from build123d import *

# Parameters (mm, degrees)
SKETCH2_W           = 37
SKETCH2_H           = 8
SKETCH2_R           = 2.1
BOSS_EXTRUDE1_DEPTH = 5
SKETCH3_W           = 37
SKETCH3_H           = 5
BOSS_EXTRUDE2_DEPTH = 6
SKETCH4_W           = 37
SKETCH4_H           = 5
BOSS_EXTRUDE3_DEPTH = 57
SKETCH5_W           = 37
SKETCH5_H           = 5
BOSS_EXTRUDE4_DEPTH = 27.5
SKETCH6_R           = 60
BOSS_EXTRUDE5_DEPTH = 5


with BuildPart() as part:
    # Sketch2 → Boss-Extrude1 (new body)
    with BuildSketch(Plane.XY.offset(-2347.018325578)):
        with Locations((0, 1)):
            Rectangle(SKETCH2_W, SKETCH2_H)
        with Locations((10, 1)):
            Circle(SKETCH2_R, mode=Mode.SUBTRACT)
        with Locations((-10, 1)):
            Circle(SKETCH2_R, mode=Mode.SUBTRACT)
    extrude(amount=BOSS_EXTRUDE1_DEPTH)

    # Sketch3 → Boss-Extrude2 (add)
    with BuildSketch(Plane(origin=(0, 5, 0), x_dir=(1, 0, 0), z_dir=(0, 1, 0))):
        with Locations((0, 2344.518325578)):
            Rectangle(SKETCH3_W, SKETCH3_H)
    extrude(amount=BOSS_EXTRUDE2_DEPTH)

    # Sketch4 → Boss-Extrude3 (add)
    with BuildSketch(Plane.XY.offset(-2342.018325578)):
        with Locations((0, 8.5)):
            Rectangle(SKETCH4_W, SKETCH4_H)
    extrude(amount=BOSS_EXTRUDE3_DEPTH)

    # Sketch5 → Boss-Extrude4 (add)
    with BuildSketch(Plane(origin=(0, 11, 0), x_dir=(1, 0, 0), z_dir=(0, 1, 0))):
        with Locations((0, 2287.518325578)):
            Rectangle(SKETCH5_W, SKETCH5_H)
    extrude(amount=BOSS_EXTRUDE4_DEPTH)

    # Sketch6 → Boss-Extrude5 (add)
    with BuildSketch(Plane.XY.offset(-2285.018325578)):
        with Locations((-0.279431791, 76.5)):
            Circle(SKETCH6_R)
    extrude(amount=-BOSS_EXTRUDE5_DEPTH)


solid = part.part
For this review, take the finished solid that the model builds, in its own axes (mm). A direction names the side the tool comes from. Round coordinates to 2 decimals unless told otherwise and drop trailing zeros. Write each loop counter-clockwise with the first axis right and the second up, starting at its lowest first coordinate (ties: lowest second). Pieces come first, ordered by that corner, then holes. Notation, with made-up numbers: (2.25, 82) -> (43.25, 82) arc R9 ccw to (43.25, 98) -> close; hole circle Ø10 at (-1, 29). An arc over 180 degrees is marked (long way). Use CSV: the item, a comma, the result in double quotes.
(1) Consider section A-A, the plane y = 1. Give the boundary of the cut face in (x, z).
Computed values:
outline,"(-18.5, -2347.02) -> (-12.1, -2347.02) -> (-12.1, -2342.02) -> (-18.5, -2342.02) -> close; (-7.9, -2347.02) -> (7.9, -2347.02) -> (7.9, -2342.02) -> (-7.9, -2342.02) -> close; (12.1, -2347.02) -> (18.5, -2347.02) -> (18.5, -2342.02) -> (12.1, -2342.02) -> close"
(2) Consider section C-C, the plane z = -2320.5. Give the boundary of the cut face in (x, y), plus the area to 3 significant figures.
Computed values:
outline,"(-18.5, 6) -> (18.5, 6) -> (18.5, 11) -> (-18.5, 11) -> close"
area,"185 mm²"
(3) Draft analysis for pull direction X (two halves, no side actions). For faces 1 (the face through (-12.1, 1.09, -2344.55)), 2 (the face through (-1, 75, -2290.018)), 3 (the face through (18.5, 9, -2316)), state which applies: +X half, -X half, draft (parallel to the pull), parting line (faces both ways), or undercut.
Computed values:
face 1,"undercut"
face 2,"draft"
face 3,"+X half"
(4) To check wall thickness, follow L1, parallel to Y at x = 10, z = -2345; L2, parallel to Y at x = -18, z = -2330; L3, parallel to Z at x = 42.5, y = 43. State the ranges of each line that lie inside material, in increasing order. Write a range as [from, to].
Computed values:
L1,"[-3, -1.1], [3.1, 11]"
L2,"[6, 11]"
L3,"[-2290.02, -2285.02]"
(5) For faces 4 (the face through (0, 6, -2314)), 5 (the face through (-18.5, 9, -2316)), 6 (the face through (0, 11, -2319)), list the 3-axis set-ups (+Z, -Z, +X, -X, +Y, -Y) from which the entire face can be reached by the end or side of a thin tool; tool diameter is ignored.
Computed values:
face 4,"+Z, +X, -X, -Y"
face 5,"+Z, -Z, -X, -Y"
face 6,"-Z, +X, -X, +Y"
(6) Consider section B-B, the plane x = 10. Give the boundary of the cut face in (y, z).
Computed values:
outline,"(-3, -2347.02) -> (-1.1, -2347.02) -> (-1.1, -2342.02) -> (-3, -2342.02) -> close; (3.1, -2347.02) -> (11, -2347.02) -> (11, -2290.02) -> (135.61, -2290.02) -> (135.61, -2285.02) -> (6, -2285.02) -> (6, -2342.02) -> (3.1, -2342.02) -> close"
(7) Clearance check with flat-ended pins moving along their axes: P1, Ø4, axis at x = -16, z = -2316.5, coming from the +Y side; P2, Ø6, axis at x = 33.5, y = 66, coming from the -Z side; P3, Ø18, axis at y = 8.5, z = -2316, coming from the +X side. State where each tip first meets the part, or that it passes through.
Computed values:
P1,"y = 11"
P2,"z = -2290.02"
P3,"x = 18.5"
(8) Consider section D-D, the plane y = 76.5. Give the boundary of the cut face in (x, z).
Computed values:
outline,"(-60.28, -2290.02) -> (59.72, -2290.02) -> (59.72, -2285.02) -> (-60.28, -2285.02) -> close"
